Autodesk Inventor part; units mm, degrees
ref_plane "YZ Plane" through (0, 0, 0) normal (1, 0, 0) x (0, 1, 0)
ref_plane "XZ Plane" through (0, 0, 0) normal (0, 1, 0) x (-1, 0, 0)
ref_plane "XY Plane" through (0, 0, 0) normal (0, 0, 1) x (1, 0, 0)
sketch "Sketch1" plane through (0, 0, 0) normal (0, 1, 0) x (-1, 0, 0)
  line L0 (153, 85) -> (0, 85)
  line L1 (0, 65) -> (-3, 65)
  line L2 (-3, 65) -> (-3, 60)
  line L3 (-3, 60) -> (0, 60)
  line L4 (0, 40) -> (153, 40) construction
  line L5 (0, 27.5) -> (-3, 27.5)
  line L6 (-3, 27.5) -> (-3, 17.5)
  line L7 (-3, 17.5) -> (0, 17.5)
  line L8 (153, 65) -> (156, 65)
  line L9 (156, 65) -> (156, 60)
  line L10 (156, 60) -> (153, 60)
  line L11 (153, 27.5) -> (156, 27.5)
  line L12 (156, 27.5) -> (156, 17.5)
  line L13 (156, 17.5) -> (153, 17.5)
  line L14 (153, 65) -> (153, 85)
  line L15 (153, 0) -> (153, 17.5)
  line L16 (153, 27.5) -> (153, 60)
  line L17 (0, 85) -> (0, 65)
  line L18 (0, 60) -> (0, 27.5)
  line L19 (0, 17.5) -> (0, 0)
  line L20 (40, 0) -> (40, -3)
  line L21 (40, -3) -> (26, -3)
  line L22 (26, -3) -> (26, 0)
  line L23 (127, 0) -> (127, -3)
  line L24 (127, -3) -> (113, -3)
  line L25 (113, -3) -> (113, 0)
  line L26 (0, 0) -> (26, 0)
  line L27 (40, 0) -> (113, 0)
  line L28 (127, 0) -> (153, 0)
  dimension "d0" = 85
  dimension "d1" = 153
  dimension "d3" = 3
  dimension "d4" = 20
  dimension "d5" = 10
  dimension "d6" = 3
  dimension "d9" = 3
  dimension "d10" = 10
  dimension "d11" = 3
  dimension "d12" = 12.5
  dimension "d13" = 20
  dimension "d16" = 20
  dimension "d39" = 14
  dimension "d40" = 3
  dimension "d41" = 14
  dimension "d42" = 3
  dimension "d43" = 26
  dimension "d44" = 26
  dimension "d64" = 12.5
  dimension "d65" = 5
  dimension "d66" = 5
extrude "Extrusion1" add sketch "Sketch1" along normal blind 3
sketch "Sketch2" plane through (0, 3, 0) normal (0, 1, 0) x (1, 0, 0)
  line L0 (-153, -27.5) -> (-153, -60)
  line L1 (0, -60) -> (0, -27.5)
  line L2 (-143, -30) -> (-135, -30)
  line L3 (-135, -60) -> (-153, -60)
  line L4 (-135, -24) -> (-132, -24)
  line L5 (-132, -66) -> (-135, -66)
  line L6 (-132, -30) -> (-112, -30)
  line L7 (-112, -30) -> (-112, -60)
  line L8 (-112, -60) -> (-132, -60)
  line L9 (-132, -24) -> (-132, -30)
  line L10 (-132, -60) -> (-132, -66)
  line L11 (-135, -66) -> (-135, -60)
  line L12 (-135, -30) -> (-135, -24)
  line L13 (-153, -60) -> (-153, -30)
  line L14 (3, -27.5) -> (3, -17.5)
  line L15 (-153, -40) -> (0, -40) construction
  line L16 (0, -27.5) -> (3, -27.5)
  line L17 (-153, -27.5) -> (-143, -27.5)
  line L18 (-143, -27.5) -> (-143, -30)
  point P0 (-156, -60)
  dimension "d22" = 42
  dimension "d24" = 3
  dimension "d26" = 6
  dimension "d29" = 41
  dimension "d67" = 20
  dimension "d68" = 10
  dimension "d69" = 20
  dimension "d70" = 6
  dimension "d109" = 10
  dimension "d154" = 2.5
extrude "Extrusion2" cut sketch "Sketch2" against normal through all
sketch "Sketch3" plane through (0, 3, 0) normal (0, 1, 0) x (1, 0, 0)
  line L0 (-153, -85) -> (0, -85)
  line L1 (0, -60) -> (0, -27.5)
  line L2 (-112, -30) -> (-112, -60)
  line L3 (-48, -37) -> (-48, -42)
  line L4 (-53, -47) -> (-75, -47)
  arc A0 (-48, -37) -> (-53, -32) centre (-53, -37) ccw
  arc A1 (-53, -47) -> (-48, -42) centre (-53, -42) ccw
  arc A2 (-80, -42) -> (-75, -47) centre (-75, -42) ccw
  line L5 (-40, 0) -> (-113, 0)
  line L6 (-75, -32) -> (-53, -32)
  line L7 (-80, -42) -> (-80, -37)
  arc A3 (-75, -32) -> (-80, -37) centre (-75, -37) ccw
  point P0 (-115, -26)
  point P1 (-115, -30)
  point P2 (-116, -20)
  point P3 (-79, 0)
  point P4 (-73, 0)
  point P5 (-112, -32)
  point P6 (-112, -26)
  dimension "d34" = 38
  dimension "d35" = 48
  dimension "d116" = 32
  dimension "d117" = 5
  dimension "d177" = 5
  dimension "d178" = 32
extrude "Extrusion3" cut sketch "Sketch3" against normal through all
sketch "Sketch6" plane through (0, 0, 0) normal (0, -1, 0) x (1, 0, 0)
  line L0 (0, 27.5) -> (0, 60)
  line L1 (-156, 60) -> (-135, 60)
  line L2 (0, 52.5) -> (-10, 52.5)
  line L3 (-10, 52.5) -> (-10, 27.5)
  line L4 (-10, 27.5) -> (0, 27.5)
  line L5 (0, 27.5) -> (0, 52.5)
  line L6 (0, 40) -> (-157, 40) construction
  point P0 (-143, 60)
  dimension "d74" = 10
  dimension "d76" = 25
  dimension "d77" = 20
  dimension "d78" = 12.5
extrude "Extrusion6" cut sketch "Sketch6" against normal through all
fillet "Fillet2" radius 2 2 edges at (-10, 1.5, 52.5) (-10, 1.5, 27.5)
fillet "Fillet4" radius 1 1 edges at (-112, 1.5, 60)
sketch "Sketch5" plane through (0, 0, 0) normal (0, -1, 0) x (1, 0, 0)
  line L0 (0, 85) -> (-153, 85)
  line L1 (-153, 85) -> (-153, 65)
  circle A0 centre (-149, 82) radius 1.5
  circle A1 centre (-149, 8) radius 1.5
  circle A2 centre (-5, 82) radius 1.5
  circle A3 centre (-29, 8) radius 1.5
  point P0 (-154, 50.75)
  dimension "d51" = 3
  dimension "d53" = 4
  dimension "d54" = 3
  dimension "d56" = 3
  dimension "d57" = 74
  dimension "d58" = 144
  dimension "d59" = 3
  dimension "d60" = 3
  dimension "d61" = 24
extrude "Extrusion8" cut sketch "Sketch5" against normal through all
fillet "Fillet10" radius 2 1 edges at (-112, 1.5, 30)
sketch "Sketch10" plane through (0, 0, 0) normal (0, -1, 0) x (1, 0, 0)
  line L0 (-130, 15) -> (-122, 15)
  line L1 (-120, 13) -> (-120, 5)
  line L2 (-122, 3) -> (-130, 3)
  line L3 (-132, 5) -> (-132, 13)
  line L4 (-153, 85) -> (-153, 65)
  line L5 (0, 85) -> (-153, 85)
  arc A0 (-132, 5) -> (-130, 3) centre (-130, 5) ccw
  arc A1 (-122, 3) -> (-120, 5) centre (-122, 5) ccw
  arc A2 (-120, 13) -> (-122, 15) centre (-122, 13) ccw
  arc A3 (-130, 15) -> (-132, 13) centre (-130, 13) ccw
  line L6 (-31, 15) -> (-23, 15)
  line L7 (-21, 13) -> (-21, 5)
  line L8 (-23, 3) -> (-31, 3)
  line L9 (-33, 5) -> (-33, 13)
  line L10 (0, 65) -> (0, 85)
  arc A4 (-31, 15) -> (-33, 13) centre (-31, 13) ccw
  arc A5 (-21, 13) -> (-23, 15) centre (-23, 13) ccw
  arc A6 (-23, 3) -> (-21, 5) centre (-23, 5) ccw
  arc A7 (-33, 5) -> (-31, 3) centre (-31, 5) ccw
  line L11 (-153, 0) -> (-127, 0)
  point P0 (0, 0)
  point P1 (-132, 15)
  point P2 (-120, 3)
  point P3 (-132, 3)
  point P4 (-21, 3)
  point P5 (-21, 15)
  point P6 (-33, 3)
  point P7 (-126, 15)
  point P8 (-27, 15)
  dimension "d135" = 12
  dimension "d136" = 12
  dimension "d137" = 21
  dimension "d139" = 2
  dimension "d142" = 12
  dimension "d143" = 12
  dimension "d145" = 21
  dimension "d146" = 2
  dimension "d155" = 3
extrude "Extrusion13" cut sketch "Sketch10" against normal through all
fillet "Fillet11" radius 1 2 edges at (-143, 1.5, 30) (-143, 1.5, 27.5)
fillet "Fillet12" radius 1 2 edges at (-132, 1.5, 66) (-132, 1.5, 24)
fillet "Fillet13" radius 0.5 2 edges at (-135, 1.5, 60) (-135, 1.5, 30)
fillet "Fillet14" radius 1 2 edges at (-135, 1.5, 24) (-135, 1.5, 66)
sketch "Sketch11" plane through (0, 0, 0) normal (0, -1, 0) x (1, 0, 0)
  line L0 (-126, 30) -> (-132, 30)
  line L1 (-132, 30) -> (-132, 27)
  line L2 (-132, 27) -> (-126, 27)
  line L3 (-126, 27) -> (-126, 30)
  line L4 (-114, 30) -> (-132, 30)
  line L5 (-132, 30) -> (-132, 25)
  line L6 (-132, 60) -> (-126, 60)
  line L7 (-126, 60) -> (-126, 63)
  line L8 (-126, 63) -> (-132, 63)
  line L9 (-132, 63) -> (-132, 60)
  line L10 (-132, 60) -> (-113, 60)
  point P0 (0, 0)
  point P1 (-130, 30)
  point P2 (-132, 28)
  point P3 (-130, 60)
  dimension "d158" = 6
  dimension "d159" = 3
  dimension "d163" = 3
extrude "Extrusion14" cut sketch "Sketch11" against normal through all
sketch "Sketch12" plane through (0, 0, 0) normal (0, -1, 0) x (1, 0, 0)
  line L0 (-105, 75) -> (-97, 75)
  line L1 (-95, 73) -> (-95, 65)
  line L2 (-97, 63) -> (-105, 63)
  line L3 (-107, 65) -> (-107, 73)
  line L4 (-107, 75) -> (-95, 63) construction
  line L5 (-95, 75) -> (-107, 63) construction
  line L6 (-153, 85) -> (-153, 65)
  line L7 (0, 85) -> (-153, 85)
  line L8 (-48, 63) -> (-56, 63)
  line L9 (-58, 65) -> (-58, 73)
  line L10 (-56, 75) -> (-48, 75)
  line L11 (-46, 73) -> (-46, 65)
  line L12 (-46, 63) -> (-58, 75) construction
  line L13 (-58, 63) -> (-46, 75) construction
  line L14 (0, 65) -> (0, 85)
  arc A0 (-105, 75) -> (-107, 73) centre (-105, 73) ccw
  arc A1 (-95, 73) -> (-97, 75) centre (-97, 73) ccw
  arc A2 (-97, 63) -> (-95, 65) centre (-97, 65) ccw
  arc A3 (-107, 65) -> (-105, 63) centre (-105, 65) ccw
  arc A4 (-56, 75) -> (-58, 73) centre (-56, 73) ccw
  arc A5 (-46, 73) -> (-48, 75) centre (-48, 73) ccw
  arc A6 (-48, 63) -> (-46, 65) centre (-48, 65) ccw
  arc A7 (-58, 65) -> (-56, 63) centre (-56, 65) ccw
  point P0 (0, 0)
  point P1 (-101, 69)
  point P2 (-52, 69)
  dimension "d166" = 52
  dimension "d167" = 16
  dimension "d168" = 12
  dimension "d169" = 12
  dimension "d170" = 16
  dimension "d171" = 52
  dimension "d172" = 12
  dimension "d173" = 12
  dimension "d174" = 2
extrude "Extrusion15" cut sketch "Sketch12" against normal through all
properties part number "MainPanelCover6"
For this review, take the finished solid that the model builds, in its own axes (mm). A direction names the side the tool comes from. Coordinates: 2 decimals unless noted, no trailing zeros. Order: outer loops, then holes, each group sorted by start corner. A loop starts at its lowest first (then second) coordinate and runs counter-clockwise, first axis right, second up. Notation, with made-up numbers: (-22, -21) -> (29, -21) arc R24 ccw to (29, -3) -> close; hole circle Ø1 at (65.5, 81.25). An arc over 180 degrees is marked (long way). Use CSV: the item, a comma, the result in double quotes. Start each with the question number.
Item 1: We need section A-A, the plane z = 8. Give the boundary of the cut face in (x, y), then the cut area to 3 significant figures.
Item 2: We need section C-C, the plane x = -149. Give the boundary of the cut face in (y, z), then the cut area to 4 significant figures.
Item 3: We need section D-D, the plane y = 1.7. Give the number of separate pieces and of enclosed holes in the cut face, then the cut area to 3 significant figures.
Item 4: Insertion check: pin 1 (0.9 mm diameter, centred on x = -80, y = 1, fed in from -Z); pin 2 (0.9 mm diameter, centred on y = 1, z = -1, fed in from -X); pin 3 (1.5 mm diameter, centred on x = 1, y = 1.5, fed in from -Z). Each pin has a flat end and moves straight along its axis. Give the tip position at first contact, or say it passes through.
Item 5: Wall thickness on probe 1 along X at (y, z) = (0.7, 82); probe 2 along Z at (x, y) = (-149, 0.65); probe 3 along X at (y, z) = (1.85, 5.5): over which ranges is each line inside the solid? List them lowest first.
Item 6: We need section B-B, the plane x = -124. Give the boundary of the cut face in (y, z), then the cut area to 3 significant figures.
Item 7: Draft analysis for pull direction Z (two halves, no side actions). For faces 1 (the face through (-78, 1, 85)), 2 (the face through (0, 1, 9)), 3 (the face through (-76, 1, 0)), 4 (the face through (-58, 1, 69)), state which applies: pulls with the +Z half, pulls with the -Z half, needs draft (parallel to the pull), parting line crosses it, or undercut.
Item 8: For faces 5 (the face through (-150, 2, 27.5)), 6 (the face through (0, 1, 75)), 7 (the face through (-10, 1, 40)), 8 (the face through (-129, 1, 27)), 9 (the face through (-127, 1, -1)), list the 3-axis set-ups (+Z, -Z, +X, -X, +Y, -Y) from which the entire face can be reached by the end or side of a thin tool; tool diameter is ignored.
Derived:
1,outline,"(-153, 0) -> (-150.5, 0) -> (-150.5, 3) -> (-153, 3) -> close; (-147.5, 0) -> (-132, 0) -> (-132, 3) -> (-147.5, 3) -> close; (-120, 0) -> (-33, 0) -> (-33, 3) -> (-120, 3) -> close; (-21, 0) -> (0, 0) -> (0, 3) -> (-21, 3) -> close"
1,area,"378 mm^2"
2,outline,"(0, 0) -> (3, 0) -> (3, 6.5) -> (0, 6.5) -> close; (0, 9.5) -> (3, 9.5) -> (3, 27.5) -> (0, 27.5) -> close; (0, 60) -> (3, 60) -> (3, 80.5) -> (0, 80.5) -> close; (0, 83.5) -> (3, 83.5) -> (3, 85) -> (0, 85) -> close"
2,area,"139.5 mm^2"
3,separate pieces,"1"
3,enclosed holes,"8"
3,area,"10,600 mm^2"
4,pin 1,"stops at z = 0"
4,pin 2,"stops at x = -127"
4,pin 3,"stops at z = 17.5"
5,probe 1,"x = -153 to -150.5, -147.5 to -6.5, -3.5 to 0"
5,probe 2,"z = 0 to 6.5, 9.5 to 27.5, 60 to 80.5, 83.5 to 85"
5,probe 3,"x = -153 to -132, -120 to -33, -21 to 0"
6,outline,"(0, -3) -> (3, -3) -> (3, 3) -> (0, 3) -> close; (0, 15) -> (3, 15) -> (3, 30) -> (0, 30) -> close; (0, 60) -> (3, 60) -> (3, 85) -> (0, 85) -> close"
6,area,"138 mm^2"
7,face 1,"pulls with the +Z half"
7,face 2,"needs draft"
7,face 3,"pulls with the -Z half"
7,face 4,"undercut"
8,face 5,"-X, +Y, -Y"
8,face 6,"+Z, +X, +Y, -Y"
8,face 7,"+X, +Y, -Y"
8,face 8,"+Y, -Y"
8,face 9,"-Z, -X, +Y, -Y"
